Design review of the part built by this model. Coordinates are the model's own, in mm. Coordinates: 2 decimals unless noted, no trailing zeros. Write each loop counter-clockwise with the first axis right and the second up, starting at its lowest first coordinate (ties: lowest second). Pieces come first, ordered by that corner, then holes. Notation, with made-up numbers: (71, 75) - (108, 75) arc R30 ccw to (108, 101) - close; hole circle Ø1 at (-5, -27). An arc over 180 degrees is marked (long way). One line per item, written item: value.
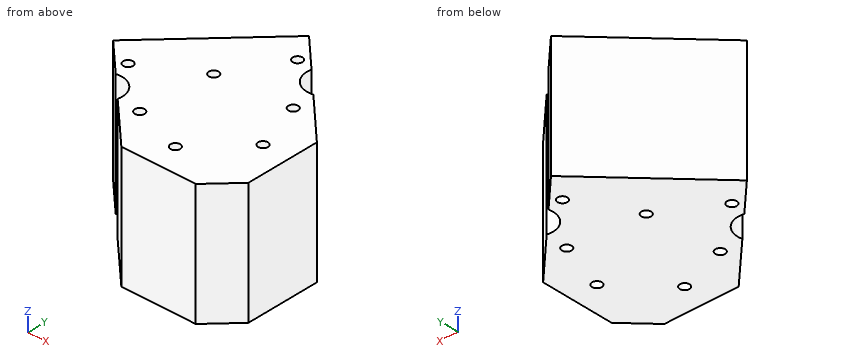
from build123d import *

# Parameters (mm, degrees)
BOSS_EXTRUDE1_DEPTH = 38.0226
SKETCH4_R           = 1.5
CUT_EXTRUDE2_DEPTH  = 133.893603459


with BuildPart() as part:
    # Sketch1 → Boss-Extrude1 (new body)
    with BuildSketch(Plane.XY):
        with BuildLine():
            Line((-58.458365937, 90.041634063), (-90.041634063, 58.458365937))
            Line((-90.041634063, 58.458365937), (-80.085733054, 48.520837101))
            ThreePointArc((-80.085733054, 48.520837101), (-74.352118178, 46.871638295), (-72.692331868, 41.141079365))
            Line((-72.692331868, 41.141079365), (-58.525108947, 27))
            Line((-58.525108947, 27), (-35.485281374, 27))
            Line((-35.485281374, 27), (-27, 35.485281374))
            Line((-27, 35.485281374), (-27, 58.525108947))
            Line((-27, 58.525108947), (-41.141079365, 72.692331868))
            ThreePointArc((-41.141079365, 72.692331868), (-46.871638295, 74.352118178), (-48.520837101, 80.085733054))
            Line((-48.520837101, 80.085733054), (-58.458365937, 90.041634063))
        make_face()
    extrude(amount=BOSS_EXTRUDE1_DEPTH)

    # Sketch4 → Cut-Extrude2 (cut, through all)
    with BuildSketch(Plane.XY.offset(38.0226)):
        with Locations((-63.639610307, 63.639610307)):
            Circle(SKETCH4_R)
        with Locations((-80.960118382, 53.639610307)):
            Circle(SKETCH4_R)
        with Locations((-53.639610307, 80.960118382)):
            Circle(SKETCH4_R)
        with Locations((-40.658639918, 65.40737726)):
            Circle(SKETCH4_R)
        with Locations((-65.40737726, 40.658639918)):
            Circle(SKETCH4_R)
        with Locations((-49.497474683, 35.355339059)):
            Circle(SKETCH4_R)
        with Locations((-35.355339059, 49.497474683)):
            Circle(SKETCH4_R)
    extrude(amount=-CUT_EXTRUDE2_DEPTH, mode=Mode.SUBTRACT)


solid = part.part
1. Consider section A-A, the plane z = 21.5. Write out the cut boundary in (x, y), then the cut area to 3 significant figures.
Answer block:
outline: (-90.04, 58.46) - (-80.09, 48.52) arc R6.17 cw to (-72.69, 41.14) - (-58.53, 27) - (-35.49, 27) - (-27, 35.49) - (-27, 58.53) - (-41.14, 72.69) arc R6.17 cw to (-48.52, 80.09) - (-58.46, 90.04) - close; hole circle Ø3 at (-80.96, 53.64); hole circle Ø3 at (-65.41, 40.66); hole circle Ø3 at (-63.64, 63.64); hole circle Ø3 at (-53.64, 80.96); hole circle Ø3 at (-49.5, 35.36); hole circle Ø3 at (-40.66, 65.41); hole circle Ø3 at (-35.36, 49.5)
area: 2,360 mm^2
2. Consider section B-B, the plane y = 46.5. Write out the cut boundary in (x, z), then the cut area to 3 significant figures.
Answer block:
outline: (-74.01, 0) - (-27, 0) - (-27, 38.02) - (-74.01, 38.02) - close
area: 1,790 mm^2
3. Wall thickness on line 1 along Y through (x, z) = (-64.5, 11); line 2 along Y through (x, z) = (-63.5, 32); line 3 along Y through (x, z) = (-53, 4): over which ranges is each line inside the solid? List them lowest first.
Answer block:
line 1: y = 32.96 to 39.46, 41.85 to 62.41, 64.87 to 84
line 2: y = 31.97 to 62.15, 65.13 to 85
line 3: y = 27 to 79.6, 82.32 to 84.57
4. Insertion check: pin 1 Ø8 at (y, z) = (69.5, 8) entering from +X; pin 2 Ø2 at (x, z) = (-80, 24) entering from +Y; pin 3 Ø1.8 at (x, y) = (-49.5, 35.36) entering from +Z; pin 4 Ø1 at (y, z) = (82, 30.5) entering from +X. Each pin has a flat end and moves straight along its axis. Give the tip position at first contact, or say it passes through.
Answer block:
pin 1: stops at x = -33.96
pin 2: stops at y = 69.5
pin 3: passes through
pin 4: stops at x = -49.93
5. Consider section C-C, the plane x = -57.5. Write out the cut boundary in (y, z), then the cut area to 3 significant figures.
Answer block:
outline: (27, 0) - (89.08, 0) - (89.08, 38.02) - (27, 38.02) - close
area: 2,360 mm^2
